Read the model definition and answer for the solid it produces. Units are mm, in the model's axes. Give positions to 0.01 mm unless a question says otherwise; leave off trailing zeros. Write each loop counter-clockwise with the first axis right and the second up, starting at its lowest first coordinate (ties: lowest second). Pieces come first, ordered by that corner, then holes. Notation, with made-up numbers: (-13, -27) -> (1, -27) arc R33 cw to (1, 9) -> close; hole circle Ø2 at (85, -28). An arc over 180 degrees is marked (long way). Put each result on its own line as item: value. Start each with the question number.
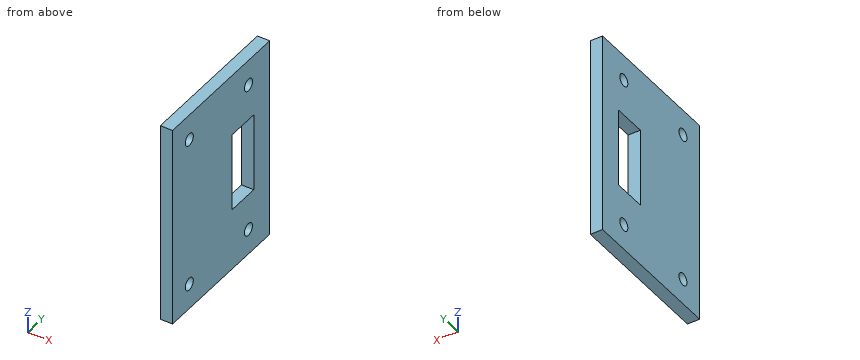
Autodesk Inventor part; units mm, degrees
ref_plane "YZ Plane" through (0, 0, 0) normal (1, 0, 0) x (0, 1, 0)
ref_plane "XZ Plane" through (0, 0, 0) normal (0, 1, 0) x (-1, 0, 0)
ref_plane "XY Plane" through (0, 0, 0) normal (0, 0, 1) x (1, 0, 0)
sketch "Sketch1" plane through (0, 0, 0) normal (1, 0, 0) x (0, 1, 0)
  line L0 (0, 0) -> (58.0898, 0)
  line L1 (58.0898, 0) -> (58.0898, -78.7908)
  line L2 (58.0898, -78.7908) -> (0, -78.7908)
  line L3 (0, -78.7908) -> (0, 0)
  dimension "d0" = 78.7908
  dimension "d1" = 58.0898
extrude "Extrusion1" add sketch "Sketch1" along normal blind 4.7752
sketch "Sketch2" plane through (4.7752, 0, 0) normal (1, 0, 0) x (0, 0, -1)
  line L0 (0, 58.0898) -> (0, 0)
  line L1 (78.7908, 58.0898) -> (0, 58.0898)
  line L2 (0, 0) -> (78.7908, 0)
  line L3 (78.7908, 0) -> (78.7908, 58.0898)
  point P0 (10, 45.3898)
  point P1 (68.7908, 45.3898)
  point P2 (10, 10)
  point P3 (68.7908, 10)
  dimension "d4" = 10
  dimension "d6" = 10
  dimension "d7" = 10
  dimension "d9" = 10
  dimension "d10" = 12.7
  dimension "d12" = 12.7
  dimension "d16" = 10
  dimension "d17" = 10
hole "Hole1" at (4.7752, 45.3898, -10) at (4.7752, 45.3898, -68.7908) at (4.7752, 10, -10) at (4.7752, 10, -68.7908) direction (-1, 0, 0) diameter 4.7752 end through all
sketch "Sketch3" plane through (4.7752, 0, 0) normal (1, 0, 0) x (0, 0, -1)
  line L0 (24.1554, 35.4838) -> (54.6354, 35.4838)
  line L1 (54.6354, 35.4838) -> (54.6354, 48.5648)
  line L2 (54.6354, 48.5648) -> (24.1554, 48.5648)
  line L3 (24.1554, 48.5648) -> (24.1554, 35.4838)
  line L4 (0, 58.0898) -> (0, 0)
  line L5 (78.7908, 58.0898) -> (0, 58.0898)
  dimension "d25" = 13.081
  dimension "d26" = 30.48
  dimension "d28" = 78.7908
  dimension "d29" = 24.1554
  dimension "d30" = 58.0898
  dimension "d31" = 9.525
extrude "Extrusion2" cut sketch "Sketch3" against normal through all
equation "\"d29\" = -0.5 * d26 + 0.5 * d28"
properties part number "SwitchBracket"
1) A cutting plane is placed at C-C on y = 38. Give the vertices of the cut face in (x, z).
2) A cutting plane is placed at D-D on x = 2.4. Give the vertices of the cut face in (y, z), and give its area (3 significant figures).
3) A cutting plane is placed at A-A on y = 10. Give the vertices of the cut face in (x, z).
4) A cutting plane is placed at B-B on z = -10. Give the vertices of the cut face in (x, y).
5) Straight lines are drawn through the part: line 1 (Y direction, x = 3.85, z = -10); line 2 (Z direction, x = 2.3, y = 10); line 3 (Y direction, x = 0.6, z = -26.5). For each, find the intervals that lie inside material, in ascending order. Write a range as [from, to].
6) This flat-tipped pin is pushed along its axis until it touches: pin 1 Ø4 at (y, z) = (10, -10) entering from -X. Where does it stop, or does it pass through?
Results found:
1. outline: (0, -78.79) -> (4.78, -78.79) -> (4.78, -54.64) -> (0, -54.64) -> close; (0, -24.16) -> (4.78, -24.16) -> (4.78, 0) -> (0, 0) -> close
2. outline: (0, -78.79) -> (58.09, -78.79) -> (58.09, 0) -> (0, 0) -> close; hole circle Ø4.78 at (10, -68.79); hole circle Ø4.78 at (10, -10); hole (35.48, -54.64) -> (48.56, -54.64) -> (48.56, -24.16) -> (35.48, -24.16) -> close; hole circle Ø4.78 at (45.39, -68.79); hole circle Ø4.78 at (45.39, -10)
2. area: 4,110 mm²
3. outline: (0, -78.79) -> (4.78, -78.79) -> (4.78, -71.18) -> (0, -71.18) -> close; (0, -66.4) -> (4.78, -66.4) -> (4.78, -12.39) -> (0, -12.39) -> close; (0, -7.61) -> (4.78, -7.61) -> (4.78, 0) -> (0, 0) -> close
4. outline: (0, 0) -> (4.78, 0) -> (4.78, 7.61) -> (0, 7.61) -> close; (0, 12.39) -> (4.78, 12.39) -> (4.78, 43) -> (0, 43) -> close; (0, 47.78) -> (4.78, 47.78) -> (4.78, 58.09) -> (0, 58.09) -> close
5. line 1: y = [0, 7.61], [12.39, 43], [47.78, 58.09]
5. line 2: z = [-78.79, -71.18], [-66.4, -12.39], [-7.61, 0]
5. line 3: y = [0, 35.48], [48.56, 58.09]
6. pin 1: passes through
